from build123d import *

# Parameters (mm, degrees)
CROQUIS1_R              = 11.375
SALIENTE_EXTRUIR1_DEPTH = 0.5
CROQUIS2_R              = 11.375
CROQUIS2_R_2            = 10.875
SALIENTE_EXTRUIR2_DEPTH = 10
REDONDEO1_R             = 0.3
REDONDEO2_R             = 0.3


with BuildPart() as part:
    # Croquis1 → Saliente-Extruir1 (new body)
    with BuildSketch(Plane(origin=(0, 0, 0), x_dir=(1, 0, 0), z_dir=(0, 1, 0))):
        with Locations(Location((0, 0, 0), (0, 0, 270))):
            Circle(CROQUIS1_R)
    extrude(amount=SALIENTE_EXTRUIR1_DEPTH)

    # Croquis2 → Saliente-Extruir2 (add)
    with BuildSketch(Plane(origin=(0, 0.5, 0), x_dir=(1, 0, 0), z_dir=(0, 1, 0))):
        with Locations(Location((0, 0, 0), (0, 0, 270))):
            Circle(CROQUIS2_R)
        with Locations(Location((0, 0, 0), (0, 0, 270))):
            Circle(CROQUIS2_R_2, mode=Mode.SUBTRACT)
    extrude(amount=SALIENTE_EXTRUIR2_DEPTH)

    # Redondeo1
    redondeo1_edges = [part.edges().sort_by_distance(p)[0] for p in [
        (0, 0.5, -10.875),
    ]]
    fillet(redondeo1_edges, radius=REDONDEO1_R)

    # Redondeo2
    redondeo2_edges = [part.edges().sort_by_distance(p)[0] for p in [
        (0, 0, -11.375),
    ]]
    fillet(redondeo2_edges, radius=REDONDEO2_R)


solid = part.part
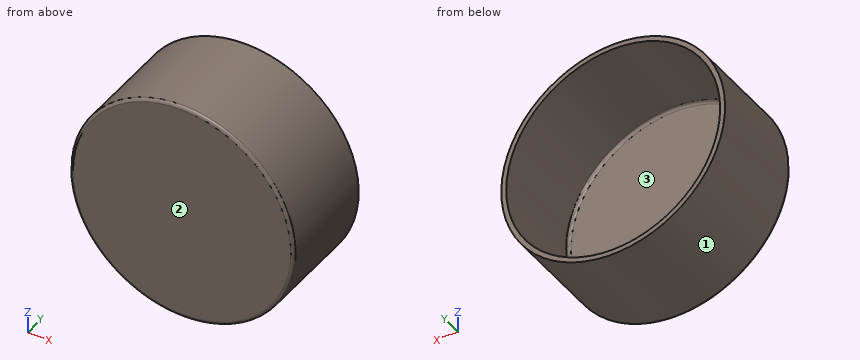
Can you work these out from the model? Positions are in its coordinate system, mm. Face numbers are marked on the shaded views. Round coordinates to 2 decimals unless told otherwise and drop trailing zeros. Loops run counter-clockwise (first coordinate to the right, second up) from the corner with the lowest first, then second, coordinate; pieces in that order, holes last. Notation, with made-up numbers: (28, -31.75) - (42, -31.75) arc R30 ccw to (42, -2.75) - close; hole circle Ø9 at (-1, 29.25). An arc over 180 degrees is marked (long way). Write item = value, one per line. Start each with the question number.
(1) If I drill on probe 1 along X at (y, z) = (5, 0) (3 decimals); probe 2 along Y at (x, z) = (9.25, 2.5); probe 3 along X at (y, z) = (2.25, 6), over which ranges is the centre line in solid material (lowest first)? Write a range as [from, to].
(2) For P1, Ø2, axis at y = 5, z = -6, coming from the -X side; P2, Ø1, axis at x = -5, y = 8.5, coming from the +Z side; P3, Ø1.5, axis at y = 7.5, z = 8.5, coming from the -X side, each with a flat end and sliding along its axis, tell me the tip position at first contact or that it passes through.
(3) If we mould it in two halves opening along X, with no side actions, what happens to the marked faces 1, 2 and 3? For each: released by +X, released by -X, zero draft, split by the parting line, or undercut.
(4) If we section it at A-A (x = 0): Please give me the cut outline in (y, z) (3 decimals), and give its area (3 significant figures).
(5) If we section it at C-C (y = 2.5): Please give me the cut outline in (x, z) (3 decimals).
(6) If we section it at B-B (z = 0): Please give me the cut outline in (x, y) (3 decimals).
Ans:
q1.probe_1 = [-11.375, -10.875], [10.875, 11.375]
q1.probe_2 = [0, 0.5]
q1.probe_3 = [-9.66, -9.07], [9.07, 9.66]
q2.P1 = -10.22
q2.P2 = 10.45
q2.P3 = -8.33
q3.face_1 = split by the parting line
q3.face_2 = zero draft
q3.face_3 = undercut
q4.outline = (0, -11.075) arc R0.3 ccw to (0.3, -11.375) - (10.5, -11.375) - (10.5, -10.875) - (0.8, -10.875) arc R0.3 cw to (0.5, -10.575) - (0.5, 10.575) arc R0.3 cw to (0.8, 10.875) - (10.5, 10.875) - (10.5, 11.375) - (0.3, 11.375) arc R0.3 ccw to (0, 11.075) - close
q4.area = 21.4 mm²
q5.outline = circle Ø22.75 at (0, 0); hole circle Ø21.75 at (0, 0)
q6.outline = (-11.375, 0.3) arc R0.3 ccw to (-11.075, 0) - (11.075, 0) arc R0.3 ccw to (11.375, 0.3) - (11.375, 10.5) - (10.875, 10.5) - (10.875, 0.8) arc R0.3 cw to (10.575, 0.5) - (-10.575, 0.5) arc R0.3 cw to (-10.875, 0.8) - (-10.875, 10.5) - (-11.375, 10.5) - close
